from build123d import *

# Parameters (mm, degrees)
F0_W      = 914.4
F0_H      = 812.8
F1_DEPTH  = 863.6
F3_DEPTH  = 838.2
F4_W      = 609.6
F4_H      = 660.4
F5_DEPTH  = 457.2
F6_W      = 660.4
F6_H      = 228.6
F7_DEPTH  = 152.4
F8_R      = 19.05
F9_DEPTH  = 228.6
F10_W     = 660.4
F10_H     = 63.5
F11_DEPTH = 609.6
F12_R     = 19.05
F13_DEPTH = 76.201
F14_R     = 76.2
F15_DEPTH = 54.6637094628
F16_R     = 101.6
F17_DEPTH = 76.201


with BuildPart() as f1:
    # F0 (on Top) → F1 (new body)
    with BuildSketch(Plane.XY):
        Rectangle(F0_W, F0_H)
    extrude(amount=F1_DEPTH)

    # F2 (on face) → F3 (cut)
    with BuildSketch(Plane.YZ.offset(457.2)):
        with BuildLine():
            Line((330.2, 63.5), (330.2, 279.4))
            ThreePointArc((330.2, 279.4), (0, 355.6), (-330.2, 279.4))
            Line((-330.2, 279.4), (-330.2, 63.5))
            Line((-330.2, 63.5), (330.2, 63.5))
        make_face()
    extrude(amount=-F3_DEPTH, mode=Mode.SUBTRACT)

    # F4 (on face) → F5 (cut)
    with BuildSketch(Plane.XY.offset(863.6)):
        with Locations((76.2, 0)):
            Rectangle(F4_W, F4_H)
    extrude(amount=-F5_DEPTH, mode=Mode.SUBTRACT)

    # F6 (on face) → F7 (cut)
    with BuildSketch(Plane.YZ.offset(-228.6)):
        with Locations((0, 520.7)):
            Rectangle(F6_W, F6_H)
    extrude(amount=-F7_DEPTH, mode=Mode.SUBTRACT)

    # F8 (on face) → F9 (cut, through all)
    with BuildSketch(Plane.XY.offset(863.6)):
        with Locations((-298.45, 0)):
            Circle(F8_R)
    extrude(amount=-F9_DEPTH, mode=Mode.SUBTRACT)

    # F10 (on face) → F11 (join, through all)
    with BuildSketch(Plane.YZ.offset(-228.6)):
        with Locations((0, 666.75)):
            Rectangle(F10_W, F10_H)
    extrude(amount=F11_DEPTH)

    # F12 (on face) → F13 (cut, through all)
    with BuildSketch(Plane.XZ.offset(-330.2)):
        with Locations((53.8625605404, 771.0824012756)):
            Circle(F12_R)
    extrude(amount=-F13_DEPTH, mode=Mode.SUBTRACT)

    # F14 (on face) → F15 (cut, through all)
    with BuildSketch(Plane.XY.offset(406.4)):
        Circle(F14_R)
    extrude(amount=-F15_DEPTH, mode=Mode.SUBTRACT)

    # F16 (on face) → F17 (cut, through all)
    with BuildSketch(Plane.YZ.offset(-381)):
        with Locations((0, 171.45)):
            Circle(F16_R)
    extrude(amount=-F17_DEPTH, mode=Mode.SUBTRACT)


solid = f1.part
CAD build for the part. Positions are in the model's coordinates, mm. A direction names the side the tool comes from. Give positions to 0.01 mm unless a question says otherwise; leave off trailing zeros. Write each loop counter-clockwise with the first axis right and the second up, starting at its lowest first coordinate (ties: lowest second). Pieces come first, ordered by that corner, then holes. Notation, with made-up numbers: (40, 1) -> (97, 1) arc R16 cw to (97, 29) -> close; hole circle Ø3 at (4.25, 37.25). An arc over 180 degrees is marked (long way). Return JSON: item names as keys, results as strings.
Item 1: Tool access for faces 1 (the flat face through (-6, 6, 0)), 2 (the flat face through (-5, 330.2, 522)), 3 (the flat face through (-228.6, -5, 782)), 4 (the flat face through (44, -330.2, 173)): list every direction of +Z, -Z, +X, -X, +Y, -Y with a clear straight run to the whole face (end or side of a thin tool).
Answer below:
{"face 1": "-Z, +X, -X, +Y, -Y", "face 2": "none", "face 3": "+Z", "face 4": "+X"}
Item 2: Band-saw the part on C-C (y = 0). List the corners of the cut face in (x, z), then the cut area to 3 significant figures.
Answer below:
{"outline": "(-457.2, 0) -> (457.2, 0) -> (457.2, 63.5) -> (-381, 63.5) -> (-381, 69.85) -> (-457.2, 69.85) -> close; (-457.2, 273.05) -> (-381, 273.05) -> (-381, 355.6) -> (-76.2, 355.6) -> (-76.2, 406.4) -> (-381, 406.4) -> (-381, 635) -> (-317.5, 635) -> (-317.5, 863.6) -> (-457.2, 863.6) -> close; (-279.4, 635) -> (381, 635) -> (381, 406.4) -> (76.2, 406.4) -> (76.2, 355.6) -> (457.2, 355.6) -> (457.2, 863.6) -> (381, 863.6) -> (381, 698.5) -> (-228.6, 698.5) -> (-228.6, 863.6) -> (-279.4, 863.6) -> close", "area": "238,000 mm2"}
Item 3: Band-saw the part on D-D (x = -333). List the corners of the cut face in (y, z), then the cut area to 3 significant figures.
Answer below:
{"outline": "(-406.4, 0) -> (406.4, 0) -> (406.4, 863.6) -> (-406.4, 863.6) -> close; hole (-330.2, 63.5) -> (330.2, 63.5) -> (330.2, 279.4) arc R753.53 ccw to (-330.2, 279.4) -> close; hole (-330.2, 406.4) -> (330.2, 406.4) -> (330.2, 635) -> (-330.2, 635) -> close", "area": "374,000 mm2"}
Item 4: Drill centre lines: probe 1 along X at (y, z) = (-72, 736); probe 2 along X at (y, z) = (275, 634); probe 3 along Z at (x, y) = (-39, 81). Where is each one in solid material? Low to high.
Answer below:
{"probe 1": "x = -457.2 to -228.6, 381 to 457.2", "probe 2": "x = -457.2 to -381, 381 to 457.2", "probe 3": "z = 0 to 63.5, 351.23 to 406.4, 635 to 698.5"}
Item 5: Band-saw the part on B-B (z = 171.45). List the corners of the cut face in (x, y).
Answer below:
{"outline": "(-457.2, -406.4) -> (457.2, -406.4) -> (457.2, -330.2) -> (-381, -330.2) -> (-381, -101.6) -> (-457.2, -101.6) -> close; (-457.2, 101.6) -> (-381, 101.6) -> (-381, 330.2) -> (457.2, 330.2) -> (457.2, 406.4) -> (-457.2, 406.4) -> close"}
Item 6: Band-saw the part on A-A (x = 0). List the corners of the cut face in (y, z).
Answer below:
{"outline": "(-406.4, 0) -> (406.4, 0) -> (406.4, 863.6) -> (330.2, 863.6) -> (330.2, 698.5) -> (-330.2, 698.5) -> (-330.2, 863.6) -> (-406.4, 863.6) -> close; hole (-330.2, 63.5) -> (330.2, 63.5) -> (330.2, 279.4) arc R753.53 ccw to (76.2, 351.74) -> (76.2, 406.4) -> (330.2, 406.4) -> (330.2, 635) -> (-330.2, 635) -> (-330.2, 406.4) -> (-76.2, 406.4) -> (-76.2, 351.74) arc R753.53 ccw to (-330.2, 279.4) -> close"}
Item 7: Drop a flat-ended pin along its axis: pin 1 (3 mm diameter, centred on x = -76.5, y = -292.5, fed in from +Z). Give the stop position or say it passes through.
Answer below:
{"pin 1": "stops at z = 698.5"}
Item 8: Two-plate mould, pull along Y, no slides. Class faces 5 (the flat face through (-6, 406.4, 426)), 6 (the flat face through (381, -5, 522)), 7 (the flat face through (-6, -406.4, 426)): +Y half, -Y half, draft (parallel to the pull), parting line (faces both ways), or undercut.
Answer below:
{"face 5": "+Y half", "face 6": "undercut", "face 7": "-Y half"}
